Autodesk Inventor part; units mm, degrees
ref_plane "YZ Plane" through (0, 0, 0) normal (1, 0, 0) x (0, 1, 0)
ref_plane "XZ Plane" through (0, 0, 0) normal (0, 1, 0) x (-1, 0, 0)
ref_plane "XY Plane" through (0, 0, 0) normal (0, 0, 1) x (1, 0, 0)
sketch "Sketch1" plane through (0, 0, 0) normal (0, 0, 1) x (1, 0, 0)
  circle A0 centre (0, 0) radius 1.25
  line L0 (0, 0) -> (20, 0) construction
  circle A1 centre (20, 0) radius 1.25
  arc A2 (1.2195, 2.1824) -> (-1.2195, -2.1824) centre (0, 0) ccw
  arc A3 (21.2195, -2.1824) -> (18.7805, 2.1824) centre (20, 0) ccw
  arc A4 (1.2195, 2.1824) -> (18.7805, 2.1824) centre (10, 17.8955) ccw
  arc A5 (-1.2195, -2.1824) -> (21.2195, -2.1824) centre (10, 17.8955) ccw
  dimension "d0" = 2.5
  dimension "d1" = 20
  dimension "d8" = 5
  dimension "d17" = 18
extrude "Extrusion1" add sketch "Sketch1" along normal blind 1.5
properties part number "linkageA_mini"
Source: CAD feature listing. Evaluate the final solid. Frame: model axes, mm. Round coordinates to 2 decimals unless told otherwise and drop trailing zeros. Loops run counter-clockwise (first coordinate to the right, second up) from the corner with the lowest first, then second, coordinate; pieces in that order, holes last.
1. Ray query, L1, parallel to X at y = -0.25, z = 1.4; L2, parallel to Y at x = -0.25, z = 0.7; L3, parallel to Y at x = 0, z = 0.4. Return the intervals inside material, ascending.
2. Contact query for a flat-ended pin moving along its axis: pin 1 (1.5 mm diameter, centred on x = 20, y = 0, fed in from +Z). Output: stop coordinate, or through.
3. Section query B-B on z = 0.95. Output: boundary loops of the cut face in (x, y).
4. Section query A-A on x = 1. Output: boundary loops of the cut face in (y, z).
5. Mould query, pull axis Y, two halves, no side actions, for faces 1 (the cylindrical face through (22.155, 1.267, 0.74)), 2 (the cylindrical face through (21.155, 0.479, 0.74)), 3 (the cylindrical face through (10.164, -5.104, 0.74)). Classes: released by +Y, released by -Y, zero draft, split by the parting line, or undercut.
6. Section query D-D on y = -2.5. Output: boundary loops of the cut face in (x, z).
7. Section query C-C on x = 20.5. Output: boundary loops of the cut face in (y, z), and give its area (3 significant figures).
Answers below:
1. L1: x = -2.49 to -1.22, 1.22 to 18.78, 21.22 to 22.49
1. L2: y = -2.69 to -1.22, 1.22 to 2.49
1. L3: y = -2.82 to -1.25, 1.25 to 2.5
2. pin 1: passes through
3. outline: (-1.22, -2.18) arc R23 ccw to (21.22, -2.18) arc R2.5 ccw to (18.78, 2.18) arc R18 cw to (1.22, 2.18) arc R2.5 ccw to start; hole circle Ø2.5 at (0, 0); hole circle Ø2.5 at (20, 0)
4. outline: (-3.27, 0) - (-0.75, 0) - (-0.75, 1.5) - (-3.27, 1.5) - close; (0.75, 0) - (2.29, 0) - (2.29, 1.5) - (0.75, 1.5) - close
5. face 1: split by the parting line
5. face 2: undercut
5. face 3: released by -Y
6. outline: (-0.63, 0) - (20.63, 0) - (20.63, 1.5) - (-0.63, 1.5) - close
7. outline: (-2.57, 0) - (-1.15, 0) - (-1.15, 1.5) - (-2.57, 1.5) - close; (1.15, 0) - (2.45, 0) - (2.45, 1.5) - (1.15, 1.5) - close
7. area: 4.09 mm2
